For this review, use the dimensioned drawing (mm, ordinates from the lowest corner) and the shaded views. A direction names the side the tool comes from. Coordinates: 2 decimals unless noted, no trailing zeros. Loops run counter-clockwise (first coordinate to the right, second up) from the corner with the lowest first, then second, coordinate; pieces in that order, holes last. Notation, with made-up numbers: M 26.25,-3 L 60.25,-3 A25 cw 60.25,30 Z; hole C 10.25,65 d11. An arc over 180 degrees is marked long. One line per item, written item: value.
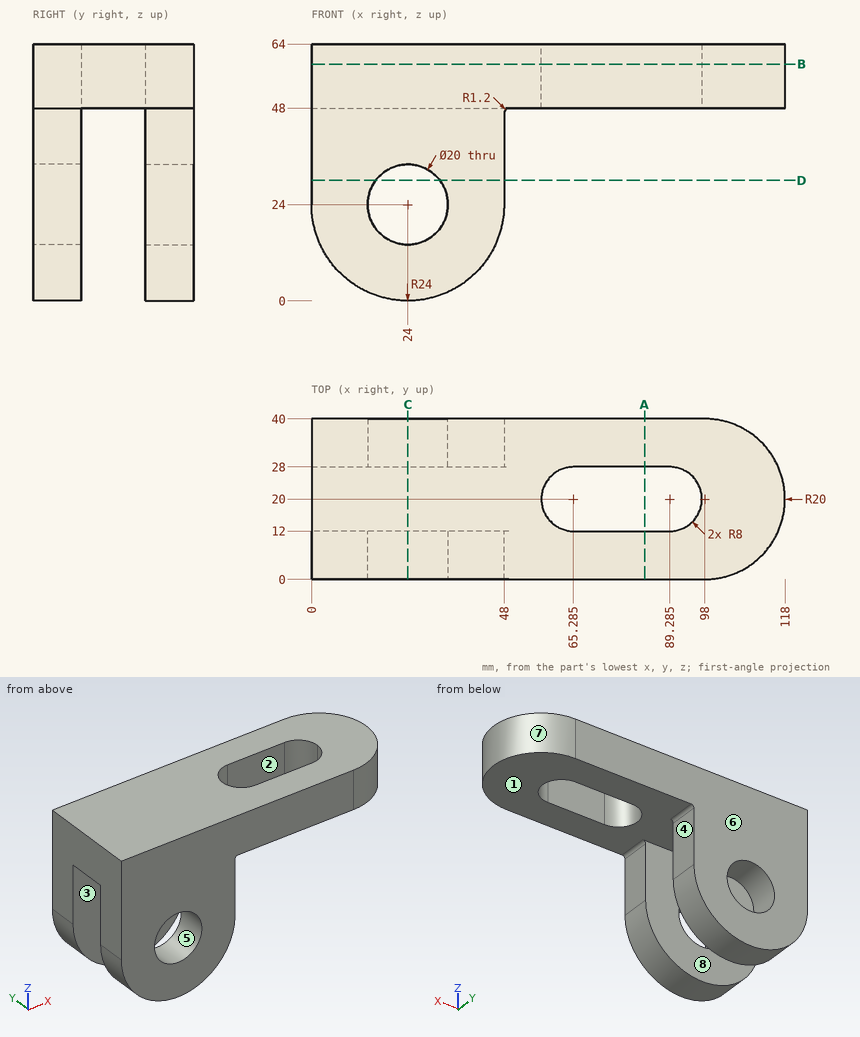
(1) Add section A-A on x = 83. State the section outline as (y, z) points.
Checks:
outline: M 0,48 L 12,48 L 12,64 L 0,64 Z; M 28,48 L 40,48 L 40,64 L 28,64 Z
(2) Insertion check: pin 1 Ø3 at (y, z) = (25.5, 52) entering from +X; pin 2 Ø9.5 at (y, z) = (35.5, 37) entering from +X; pin 3 Ø1 at (y, z) = (33.5, 7) entering from +X; pin 4 Ø8 at (y, z) = (17.5, 24) entering from +X. Each pin has a flat end and moves straight along its axis. Give the tip position at first contact, or say it passes through.
Checks:
pin 1: x = 117.6
pin 2: x = 48
pin 3: x = 41.43
pin 4: through
(3) Add section C-C on x = 24. State the section outline as (y, z) points, then the cut area to 3 significant figures.
Checks:
outline: M 0,0 L 12,0 L 12,14 L 0,14 Z; M 0,34 L 12,34 L 12,48 L 28,48 L 28,34 L 40,34 L 40,64 L 0,64 Z; M 28,0 L 40,0 L 40,14 L 28,14 Z
area: 1,310 mm^2
(4) To check wall thickness, follow L1, parallel to Z at x = 24, y = 6.25; L2, parallel to Y at x = 28, z = 39.5; L3, parallel to X at y = 5, z = 24. State the ranges of each line that lie inside material, in increasing order. Write a range as [from, to].
Checks:
L1: [0, 14], [34, 64]
L2: [0, 12], [28, 40]
L3: [0, 14], [34, 48]
(5) Draft analysis for pull direction Y (two halves, no side actions). For the marked faces 5, 6, 7 and 8, state which applies: pulls with the +Y half, pulls with the -Y half, needs draft (parallel to the pull), parting line crosses it, or undercut.
Checks:
face 5: needs draft
face 6: pulls with the +Y half
face 7: parting line crosses it
face 8: undercut
(6) Add section B-B on z = 59. State the section outline as (x, y) points (3 decimals).
Checks:
outline: M 0,0 L 98,0 A20 ccw 98,40 L 0,40 Z; hole M 65.285,12 L 89.285,12 A8 ccw 89.285,28 L 65.285,28 A8 ccw Z
(7) Tool access review of the marked faces 1, 2, 3 and 4: name each direction out of +Z, -Z, +X, -X, +Y, -Y from which nothing blocks a thin tool from reaching the whole face with its end or side.
Checks:
face 1: -Z, +X
face 2: +Z, -Z
face 3: -Z, +X, -X
face 4: -Z, +X, +Y, -Y
(8) Add section D-D on z = 30. State the section outline as (x, y) points.
Checks:
outline: M 0,0 L 16,0 L 16,12 L 0,12 Z; M 0,28 L 16,28 L 16,40 L 0,40 Z; M 32,0 L 48,0 L 48,12 L 32,12 Z; M 32,28 L 48,28 L 48,40 L 32,40 Z
